Work out the finished part from the listing and answer in its coordinate system (mm). Face numbers are marked on the shaded views. A direction names the side the tool comes from. Give positions to 0.01 mm unless a question says otherwise; leave off trailing zeros. Write each loop counter-clockwise with the first axis right and the second up, starting at its lowest first coordinate (ties: lowest second). Pieces come first, ordered by that corner, then holes. Notation, with made-up numbers: (23.25, 71.5) - (35.25, 71.5) arc R21 cw to (35.25, 75.5) - close; hole circle Ø9 at (-15.75, 41.5). An arc over 180 degrees is marked (long way). Write each question's results on one line, items separated by ' | '. Start each with the question number.
from build123d import *

# Parameters (mm, degrees)
SKETCH1_W                = 50.8
SKETCH1_H                = 50.8
SKETCH1_W_2              = 44.45
SKETCH1_H_2              = 44.45
BOSS_EXTRUDE1_DEPTH      = 304.8
BOSS_EXTRUDE2_DEPTH      = 7.9375
BOSS_EXTRUDE2_DEPTH_BACK = 89.69375
SKETCH2_W                = 50.8254
SKETCH2_H                = 50.8
SKETCH2_W_2              = 44.4754
SKETCH2_H_2              = 44.45
CUT_EXTRUDE1_DEPTH       = 371.251267642
FILLET1_R                = 4.7625
CUT_EXTRUDE2_START       = 304.7873
SKETCH1_3_W              = 44.45
SKETCH1_3_H              = 44.45
CUT_EXTRUDE2_DEPTH       = 3.175
FILLET3_R                = 4.7625


with BuildPart() as part:
    # Sketch1 → Boss-Extrude1 (new body)
    with BuildSketch(Plane(origin=(0, 0, 0), x_dir=(0, 0, -1), z_dir=(1, 0, 0))):
        with Locations((25.4, 0)):
            Rectangle(SKETCH1_W, SKETCH1_H)
        with Locations((25.4, 0)):
            Rectangle(SKETCH1_W_2, SKETCH1_H_2, mode=Mode.SUBTRACT)
    extrude(amount=BOSS_EXTRUDE1_DEPTH)

    # Sketch2 → Boss-Extrude2 (add, two sides: drawn at the far end of the back side and taken through both)
    with BuildSketch(Plane.XY.offset(-BOSS_EXTRUDE2_DEPTH_BACK)):
        with Locations((330.2, 0)):
            Rectangle(SKETCH2_W, SKETCH2_H)
        with Locations((330.2, 0)):
            Rectangle(SKETCH2_W_2, SKETCH2_H_2, mode=Mode.SUBTRACT)
    extrude(amount=BOSS_EXTRUDE2_DEPTH + BOSS_EXTRUDE2_DEPTH_BACK)

    # Sketch3 → Cut-Extrude1 (cut, through all)
    with BuildSketch(Plane(origin=(0, 25.4, 0), x_dir=(1, 0, 0), z_dir=(0, 1, 0))):
        Polygon((304.7873, 89.69375), (355.6127, 88.10625), (355.6127, 89.69375), align=None)
        Polygon((304.7873, -7.9375), (355.6127, -7.14375), (355.6127, -7.9375), align=None)
    extrude(amount=-CUT_EXTRUDE1_DEPTH, mode=Mode.SUBTRACT)

    # Fillet1
    fillet1_edges = [part.edges().sort_by_distance(p)[0] for p in [
        (152.39365, -25.4, 0),
        (152.39365, 25.4, 0),
        (152.39365, 25.4, -50.8),
        (152.39365, -25.4, -50.8),
        (304.7873, -25.4, -70.246875),
        (304.7873, -25.4, 3.96875),
        (304.7873, 25.4, -70.246875),
        (304.7873, 25.4, 3.96875),
        (355.6127, 25.4, -40.48125),
        (355.6127, -25.4, -40.48125),
    ]]
    fillet(fillet1_edges, radius=FILLET1_R)

    # Sketch1<3> → Cut-Extrude2 (cut)
    with BuildSketch(Plane(origin=(0, 0, 0), x_dir=(0, 0, -1), z_dir=(1, 0, 0)).offset(CUT_EXTRUDE2_START)):
        with Locations((25.4, 0)):
            Rectangle(SKETCH1_3_W, SKETCH1_3_H)
    extrude(amount=CUT_EXTRUDE2_DEPTH, mode=Mode.SUBTRACT)

    # Fillet3
    fillet3_edges = [part.edges().sort_by_distance(p)[0] for p in [
        (307.9623, 22.225, 2.356457709),
        (307.9623, -22.225, 2.356457709),
        (153.98115, -22.225, -47.625),
        (153.98115, 22.225, -47.625),
        (153.98115, 22.225, -3.175),
        (153.98115, -22.225, -3.175),
        (307.9623, -22.225, -68.609790417),
        (352.4377, -22.225, -40.506042291),
        (352.4377, 22.225, -40.506042291),
        (307.9623, 22.225, -68.609790417),
    ]]
    fillet(fillet3_edges, radius=FILLET3_R)


solid = part.part
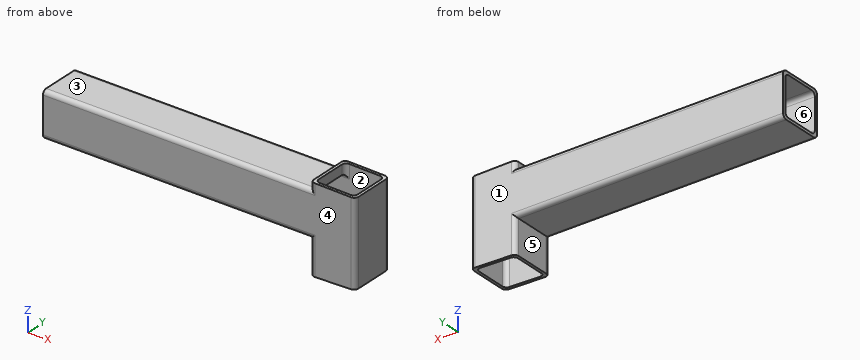
Q1. Consider L1, parallel to X at y = 2, z = -68; L2, parallel to Z at x = 147, y = 10.5 (3 decimals); L3, parallel to Y at x = 81.5, z = -10 (3 decimals). Determine where each line is inside the solid, lowest interval first.
Q2. A cutting plane is placed at A-A, the plane x = 49.5. Write down the section's boundary in (y, z) (1 decimal), and give its area (3 significant figures).
Q3. A cutting plane is placed at D-D, the plane z = -39.5. Write down the section's boundary in (x, y) (1 decimal), and give its area (3 significant figures).
Q4. A cutting plane is placed at B-B, the plane y = -3. Write down the section's boundary in (x, z) (1 decimal), and give its area (3 significant figures).
Q5. A tool of negligible diameter and unlimited length cuts with its end or side. For the marked faces 4, 5 and 6, from which of +Z, -Z, +X, -X, +Y, -Y can it reach the whole face along a straight path? Write none if from no direction.
Q6. A cutting plane is placed at C-C, the plane z = -61. Write down the section's boundary in (x, y) (1 decimal), and give its area (3 significant figures).
Q7. Given pin 1 (8.5 mm diameter, centred on y = -2, z = 5, fed in from -X); pin 2 (2 mm diameter, centred on y = 2.5, z = -2, fed in from -X); pin 3 (10.5 mm diameter, centred on x = 210, y = 0, fed in from -Z), each flat-ended and moving along its own axis, determine where each tip first touches the part or whether it passes through.
Q8. The mould has two halves that part along Z. Classify the marked faces 1, 2 and 3: pulls with the +Z half, pulls with the -Z half, needs draft (parallel to the pull), parting line crosses it, or undercut.
Result:
1) L1: x = 304.79 to 307.96, 352.44 to 355.61 | L2: z = -50.8 to -47.625, -3.175 to 0 | L3: y = -25.4 to -22.225, 22.225 to 25.4
2) outline: (-25.4, -46) arc R4.8 ccw to (-20.6, -50.8) - (20.6, -50.8) arc R4.8 ccw to (25.4, -46) - (25.4, -4.8) arc R4.8 ccw to (20.6, 0) - (-20.6, 0) arc R4.8 ccw to (-25.4, -4.8) - close; hole (-22.2, -42.9) arc R4.8 ccw to (-17.5, -47.6) - (17.5, -47.6) arc R4.8 ccw to (22.2, -42.9) - (22.2, -7.9) arc R4.8 ccw to (17.5, -3.2) - (-17.5, -3.2) arc R4.8 ccw to (-22.2, -7.9) - close | area: 605 mm2
3) outline: (0, -25.4) - (350.9, -25.4) arc R4.8 ccw to (355.6, -20.6) - (355.6, 20.6) arc R4.8 ccw to (350.9, 25.4) - (0, 25.4) - (0, 22.2) - (347.7, 22.2) arc R4.8 cw to (352.4, 17.5) - (352.4, -17.5) arc R4.8 cw to (347.7, -22.2) - (0, -22.2) - close | area: 2,400 mm2
4) outline: (0, -50.8) - (304.8, -50.8) - (304.8, -89.7) - (308, -89.6) - (308, -47.6) - (0, -47.6) - close; (0, -3.2) - (308, -3.2) - (308, 7.9) - (304.8, 7.9) - (304.8, 0) - (0, 0) - close; (352.4, -88.2) - (355.6, -88.1) - (355.6, 7.1) - (352.4, 7.2) - close | area: 2,410 mm2
5) face 4: +Z, -Z, +X, -X, -Y | face 5: -Z, -X, +Y, -Y | face 6: none
6) outline: (304.8, -20.6) arc R4.8 ccw to (309.5, -25.4) - (350.9, -25.4) arc R4.8 ccw to (355.6, -20.6) - (355.6, 20.6) arc R4.8 ccw to (350.9, 25.4) - (309.5, 25.4) arc R4.8 ccw to (304.8, 20.6) - close; hole (308, -17.5) arc R4.8 ccw to (312.7, -22.2) - (347.7, -22.2) arc R4.8 ccw to (352.4, -17.5) - (352.4, 17.5) arc R4.8 ccw to (347.7, 22.2) - (312.7, 22.2) arc R4.8 ccw to (308, 17.5) - close | area: 605 mm2
7) pin 1: stops at x = 304.79 | pin 2: stops at x = 0 | pin 3: stops at z = -50.8
8) face 1: needs draft | face 2: undercut | face 3: pulls with the +Z half
